Could you check a few things on this model? Use its own coordinates, in mm. Give positions to 0.01 mm unless a question says otherwise; leave off trailing zeros. Loops run counter-clockwise (first coordinate to the right, second up) from the corner with the lowest first, then second, coordinate; pieces in that order, holes last. Notation, with made-up numbers: M -33,-17.5 L 6,-17.5 A22 cw 6,-0.5 Z; hole C 54,-13 d7. An arc over 180 degrees is marked long. Answer in a Markdown table with one row per item. Add a question column.
1. If we section it at B-B on y = 108.5: List the corners of the cut face in (x, z) for me.
2. If we section it at D-D on z = 51.5: List the corners of the cut face in (x, y) for me.
3. I need wall thicknesses on line 1 along Y through (x, z) = (1.25, 53); line 2 along Z through (x, y) = (-2.25, 167); line 3 along Z through (x, y) = (3, 159.5). Which ranges of each line are inside material? Lowest first, please. Write a range as from..to.
4. If we section it at C-C on y = 123: List the corners of the cut face in (x, z) for me.
5. I'm going to push flat-ended pins straight in: pin 1 Ø2 at (x, z) = (-1.5, 90.5) entering from -Y; pin 2 Ø3 at (y, z) = (124.5, 4.5) entering from -X. Where does each tip first touch, or does it pass through?
6. If we section it at A-A on z = 13.5: List the corners of the cut face in (x, y) for me.
```python
from build123d import *

# Parameters (mm, degrees)
BOSS_EXTRUDE1_DEPTH      = 101.6
BOSS_EXTRUDE2_REACH      = 145.704
BOSS_EXTRUDE2_END_RADIUS = 184.15
BOSS_EXTRUDE3_REACH      = 145.81
BOSS_EXTRUDE3_END_RADIUS = 184.15


with BuildPart() as part:
    # Sketch1 → Boss-Extrude1 (new body)
    with BuildSketch(Plane.XY):
        with BuildLine():
            Line((0, 82.55), (0, 184.15))
            ThreePointArc((0, 184.15), (1.606991512, 184.142988132), (3.213860645, 184.121953063))
            Line((3.213860645, 184.121953063), (1.440696151, 82.537427235))
            ThreePointArc((1.440696151, 82.537427235), (0.720375505, 82.546856749), (0, 82.55))
        make_face()
    extrude(amount=BOSS_EXTRUDE1_DEPTH)

    # Boss-Extrude2: up to this cylinder (the profile starts inside it)
    boss_extrude2_end = Plane(origin=(0, 0, 50.8), z_dir=(0, 0, -1)) * Cylinder(BOSS_EXTRUDE2_END_RADIUS, 736.908, mode=Mode.PRIVATE)
    # Sketch2 → Boss-Extrude2 (add, up to the surface)
    with BuildSketch(Plane(origin=(1.440696151, 82.537427235, 0), x_dir=(0, 0, -1), z_dir=(-0.017452406437283546, -0.9998476951563914, 0)), mode=Mode.PRIVATE) as boss_extrude2_sk1:
        Polygon((-92.000208065, 0), (-93.4085, 2.794), (-84.3915, 2.794), (-85.799791935, 0), align=None)
    boss_extrude2_tool1 = extrude(boss_extrude2_sk1.sketch, amount=-BOSS_EXTRUDE2_REACH, mode=Mode.PRIVATE) & boss_extrude2_end
    add(boss_extrude2_tool1.solids().sort_by_distance((2.92366, 82.511542, 88.9))[0])
    # Sketch2 → Boss-Extrude2 (add, up to the surface)
    with BuildSketch(Plane(origin=(1.440696151, 82.537427235, 0), x_dir=(0, 0, -1), z_dir=(-0.017452406437283546, -0.9998476951563914, 0)), mode=Mode.PRIVATE) as boss_extrude2_sk2:
        Polygon((-15.800208065, 0), (-9.599791935, 0), (-8.1915, 2.794), (-17.2085, 2.794), align=None)
    boss_extrude2_tool2 = extrude(boss_extrude2_sk2.sketch, amount=-BOSS_EXTRUDE2_REACH, mode=Mode.PRIVATE) & boss_extrude2_end
    add(boss_extrude2_tool2.solids().sort_by_distance((2.92366, 82.511542, 12.7))[0])

    # Boss-Extrude3: up to this cylinder (the profile starts inside it)
    boss_extrude3_end = Plane(origin=(0, 0, 50.8), z_dir=(0, 0, -1)) * Cylinder(BOSS_EXTRUDE3_END_RADIUS, 737.12, mode=Mode.PRIVATE)
    # Sketch3 → Boss-Extrude3 (add, up to the surface)
    with BuildSketch(Plane(origin=(0, 82.55, 0), x_dir=(0, 0, -1), z_dir=(0, -1, 0)), mode=Mode.PRIVATE) as boss_extrude3_sk1:
        Polygon((-92.000208065, 0), (-93.4085, -2.79357446), (-84.3915, -2.79357446), (-85.799791935, 0), align=None)
    boss_extrude3_tool1 = extrude(boss_extrude3_sk1.sketch, amount=-BOSS_EXTRUDE3_REACH, mode=Mode.PRIVATE) & boss_extrude3_end
    add(boss_extrude3_tool1.solids().sort_by_distance((-1.482964, 82.55, 88.9))[0])
    # Sketch3 → Boss-Extrude3 (add, up to the surface)
    with BuildSketch(Plane(origin=(0, 82.55, 0), x_dir=(0, 0, -1), z_dir=(0, -1, 0)), mode=Mode.PRIVATE) as boss_extrude3_sk2:
        Polygon((-15.800208065, 0), (-9.599791935, 0), (-8.1915, -2.79357446), (-17.2085, -2.79357446), align=None)
    boss_extrude3_tool2 = extrude(boss_extrude3_sk2.sketch, amount=-BOSS_EXTRUDE3_REACH, mode=Mode.PRIVATE) & boss_extrude3_end
    add(boss_extrude3_tool2.solids().sort_by_distance((-1.482964, 82.55, 12.7))[0])


solid = part.part
```
Results:
| question | item | result |
|---|---|---|
| 1 | outline | M -2.79,8.19 L 0,9.6 L 0,0 L 1.89,0 L 1.89,9.6 L 4.69,8.19 L 4.69,17.21 L 1.89,15.8 L 1.89,85.8 L 4.69,84.39 L 4.69,93.41 L 1.89,92 L 1.89,101.6 L 0,101.6 L 0,92 L -2.79,93.41 L -2.79,84.39 L 0,85.8 L 0,15.8 L -2.79,17.21 Z |
| 2 | outline | M 0,82.55 A82.55 cw 1.44,82.54 L 3.21,184.12 A184.15 ccw 0,184.15 Z |
| 3 | line 1 | 82.54..184.15 |
| 3 | line 2 | 8.47..16.93, 84.67..93.13 |
| 3 | line 3 | 9.49..15.91, 85.69..92.11 |
| 4 | outline | M -2.79,8.19 L 0,9.6 L 0,0 L 2.15,0 L 2.15,9.6 L 4.94,8.19 L 4.94,17.21 L 2.15,15.8 L 2.15,85.8 L 4.94,84.39 L 4.94,93.41 L 2.15,92 L 2.15,101.6 L 0,101.6 L 0,92 L -2.79,93.41 L -2.79,84.39 L 0,85.8 L 0,15.8 L -2.79,17.21 Z |
| 5 | pin 1 | y = 82.55 |
| 5 | pin 2 | x = 0 |
| 6 | outline | M -2.79,82.55 L 0,82.55 A82.55 cw 1.44,82.54 L 4.23,82.49 L 6.01,184.05 A184.15 ccw 3.21,184.12 A184.15 ccw 0,184.15 A184.15 ccw -2.79,184.13 Z |
